Source: CAD feature listing. Evaluate the final solid. Frame: model axes, mm. A direction names the side the tool comes from. Give positions to 0.01 mm unless a question says otherwise; leave off trailing zeros. Order: outer loops, then holes, each group sorted by start corner. A loop starts at its lowest first (then second) coordinate and runs counter-clockwise, first axis right, second up.
1) Material intervals for line 1 (Y direction, x = 15.3, z = 1); line 2 (Y direction, x = 45.72, z = 0.55); line 3 (Y direction, x = -36.8, z = 0.9), sorted ascending.
2) Section D-D, the plane x = 15.3. Return loops of the section in (y, z), plus the area to 3 significant figures.
3) Section A-A, the plane x = 45.72. Return loops of the section in (y, z), plus the area to 3 significant figures.
4) Section C-C, the plane z = -7. Return loops of the section in (x, y) (3 decimals), plus the area to 3 significant figures.
5) Access query for faces 1 (the face through (-54, -11, 0)), 2 (the face through (3.7, -2.83, -6.9)), 3 (the face through (-52.705, 19, -5)). Directions: +Z, -Z, +X, -X, +Y, -Y. A direction counts if a zero-diameter tool reaches every point of the face in a straight line with its end or side. Return the directions, or none.
6) First-contact query: P1, Ø3.5, axis at x = -51, z = -3.5, coming from the +Y side (3 decimals); P2, Ø3.5, axis at x = -52, z = -8, coming from the -Y side (3 decimals); P3, Ø2, axis at x = -52, y = 21, coming from the +Z side. Flat tips, straight axial feed; report the tip coordinate or a pass-through.
7) Section B-B, the plane y = -24.25. Return loops of the section in (x, z), plus the area to 3 significant figures.
8) Draft query along Y for faces 4 (the face through (-52, 19, 0)), 5 (the face through (-35.721, -22.564, 0.811)), 6 (the face through (-49, -17.065, -5)). Return one class per face: released by +Y, released by -Y, zero draft, split by the parting line, or undercut.
```python
from build123d import *

# Parameters (mm, degrees)
SKETCH1_W            = 101.6
SKETCH1_H            = 53.5
BOSS_EXTRUDE1_DEPTH  = 1.6
M3_CLEARANCE_HOLE1_D = 3.4
SKETCH5_W            = 15.875
SKETCH5_H            = 11.43
BOSS_EXTRUDE2_DEPTH  = 10.9
SKETCH6_W            = 13.335
SKETCH6_H            = 8.89
BOSS_EXTRUDE3_DEPTH  = 10.9
SKETCH7_R            = 4.658430909
BOSS_EXTRUDE4_DEPTH  = 14


with BuildPart() as part:
    # Sketch1 → Boss-Extrude1 (new body)
    with BuildSketch(Plane.XY):
        Rectangle(SKETCH1_W, SKETCH1_H)
    extrude(amount=BOSS_EXTRUDE1_DEPTH)

    # M3 Clearance Hole1 (through all)
    with Locations(Plane(origin=(0, 0, 0), x_dir=(-1, 0, 0), z_dir=(0, 0, -1))):
        with Locations((-15.3, 19.15), (-45.72, 24.25), (-15.3, -8.75), (-39.4, -24.25), (35.5, -24.25), (36.8, 24.25)):
            Hole(M3_CLEARANCE_HOLE1_D / 2)

    # Sketch5 → Boss-Extrude2 (add)
    with BuildSketch(Plane(origin=(0, 0, 0), x_dir=(-1, 0, 0), z_dir=(0, 0, -1))):
        with Locations((49.2125, -11.35)):
            Rectangle(SKETCH5_W, SKETCH5_H)
    extrude(amount=BOSS_EXTRUDE2_DEPTH)

    # Sketch6 → Boss-Extrude3 (add)
    with BuildSketch(Plane(origin=(0, 0, 0), x_dir=(-1, 0, 0), z_dir=(0, 0, -1))):
        with Locations((46.0375, 19.13)):
            Rectangle(SKETCH6_W, SKETCH6_H)
    extrude(amount=BOSS_EXTRUDE3_DEPTH)

    # Sketch7 → Boss-Extrude4 (add)
    with BuildSketch(Plane(origin=(0, 0, 0), x_dir=(-1, 0, 0), z_dir=(0, 0, -1))):
        Circle(SKETCH7_R)
    extrude(amount=BOSS_EXTRUDE4_DEPTH)


solid = part.part
```
From the geometry:
1. line 1: y = -26.75 to -10.45, -7.05 to 17.45, 20.85 to 26.75
1. line 2: y = -26.75 to 22.55, 25.95 to 26.75
1. line 3: y = -26.75 to -25.35, -23.15 to 22.55, 25.95 to 26.75
2. outline: (-26.75, 0) - (-10.45, 0) - (-10.45, 1.6) - (-26.75, 1.6) - close; (-7.05, 0) - (17.45, 0) - (17.45, 1.6) - (-7.05, 1.6) - close; (20.85, 0) - (26.75, 0) - (26.75, 1.6) - (20.85, 1.6) - close
2. area: 74.7 mm2
3. outline: (-26.75, 0) - (22.55, 0) - (22.55, 1.6) - (-26.75, 1.6) - close; (25.95, 0) - (26.75, 0) - (26.75, 1.6) - (25.95, 1.6) - close
3. area: 80.2 mm2
4. outline: (-57.15, -17.065) - (-41.275, -17.065) - (-41.275, -5.635) - (-57.15, -5.635) - close; (-52.705, 14.685) - (-39.37, 14.685) - (-39.37, 23.575) - (-52.705, 23.575) - close; circle Ø9.317 at (0, 0)
4. area: 368 mm2
5. face 1: +Z, -X, +Y, -Y
5. face 2: -Z
5. face 3: +Z, -Z, -X, +Y
6. P1: stops at y = 23.575
6. P2: stops at y = -17.065
6. P3: stops at z = 0
7. outline: (-50.8, 0) - (-37.2, 0) - (-37.2, 1.6) - (-50.8, 1.6) - close; (-33.8, 0) - (37.7, 0) - (37.7, 1.6) - (-33.8, 1.6) - close; (41.1, 0) - (50.8, 0) - (50.8, 1.6) - (41.1, 1.6) - close
7. area: 152 mm2
8. face 4: zero draft
8. face 5: undercut
8. face 6: released by -Y
